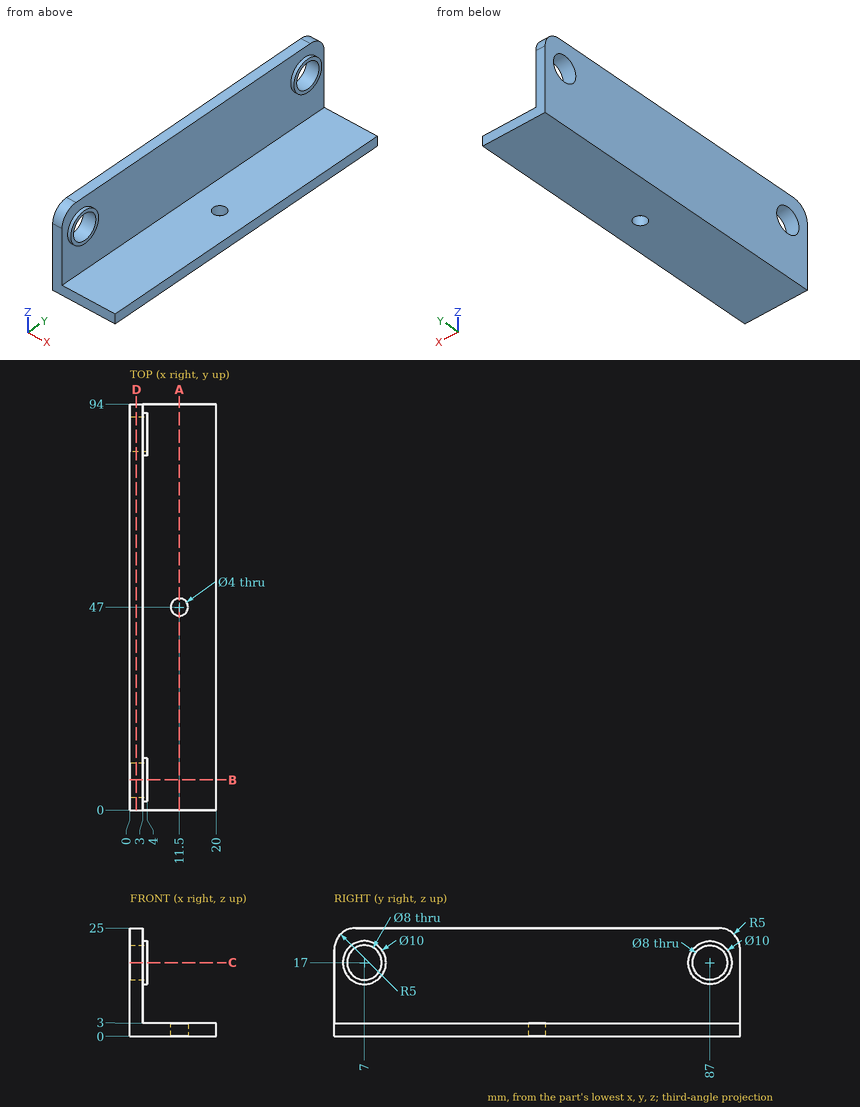
Verification items for this drawing (mm, ordinates from the low corner). Give positions to 0.01 mm unless a question says otherwise; leave off trailing zeros. Write each loop counter-clockwise with the first axis right and the second up, starting at its lowest first coordinate (ties: lowest second). Pieces come first, ordered by that corner, then holes.
1) Cross-section at C-C (z = 17). Record the boundary of the cut face in (x, y), plus the area to 3 significant figures.
Values follow:
outline: (0, 0) - (3, 0) - (3, 2) - (4, 2) - (4, 3) - (0, 3) - close; (0, 11) - (4, 11) - (4, 12) - (3, 12) - (3, 82) - (4, 82) - (4, 83) - (0, 83) - close; (0, 91) - (4, 91) - (4, 92) - (3, 92) - (3, 94) - (0, 94) - close
area: 238 mm2
2) Cross-section at B-B (y = 7). Record the boundary of the cut face in (x, z), plus the area to 3 significant figures.
Values follow:
outline: (0, 0) - (20, 0) - (20, 3) - (3, 3) - (3, 12) - (4, 12) - (4, 13) - (0, 13) - close; (0, 21) - (4, 21) - (4, 22) - (3, 22) - (3, 25) - (0, 25) - close
area: 104 mm2
3) Cross-section at D-D (x = 1.5). Record the boundary of the cut face in (y, z).
Values follow:
outline: (0, 0) - (94, 0) - (94, 20) arc R5 ccw to (89, 25) - (5, 25) arc R5 ccw to (0, 20) - close; hole circle Ø8 at (7, 17); hole circle Ø8 at (87, 17)
4) Thickness scan on line 1 (Z direction, x = 1.55, y = 7); line 2 (Z direction, x = 6, y = 43.5). Record the ranges inside material, lowest first.
Values follow:
line 1: z = 0 to 13, 21 to 25
line 2: z = 0 to 3
5) Cross-section at A-A (x = 11.5). Record the boundary of the cut face in (y, z), plus the area to 3 significant figures.
Values follow:
outline: (0, 0) - (45, 0) - (45, 3) - (0, 3) - close; (49, 0) - (94, 0) - (94, 3) - (49, 3) - close
area: 270 mm2
6) Go/stop test with flat-tipped pins: pin 1 Ø11 at (y, z) = (8, 17) entering from +X; pin 2 Ø4 at (y, z) = (15.5, 5.5) entering from +X; pin 3 Ø4 at (x, y) = (6.5, 67) entering from +Z; pin 4 Ø3 at (x, y) = (11.5, 47) entering from +Z. Record where each tip stops, or that it passes through.
Values follow:
pin 1: stops at x = 4
pin 2: stops at x = 3
pin 3: stops at z = 3
pin 4: passes through
